Geometry: final body of the model. Coordinates: model frame, mm. A direction names the side the tool comes from. Coordinates: 2 decimals unless noted, no trailing zeros. Order: outer loops, then holes, each group sorted by start corner. A loop starts at its lowest first (then second) coordinate and runs counter-clockwise, first axis right, second up. Notation, with made-up numbers: (54, -32.5) - (111, -32.5) arc R28 cw to (111, -2.5) - close; hole circle Ø5 at (66, 39.25). An arc over 180 degrees is marked (long way). Use a Markdown table: item, result. Add a question column.
```python
from build123d import *

# Parameters (mm, degrees)
SKETCH1_W           = 160
SKETCH1_H           = 120
BOSS_EXTRUDE1_DEPTH = 3
SKETCH2_W           = 160
SKETCH2_H           = 120
SKETCH2_W_2         = 148
SKETCH2_H_2         = 116
BOSS_EXTRUDE2_DEPTH = 50
SKETCH3_R           = 1
CUT_EXTRUDE1_DEPTH  = 179.910592196
SKETCH4_R           = 1.6
SKETCH4_R_2         = 2.6
SKETCH4_R_3         = 1.4
CUT_EXTRUDE2_DEPTH  = 173.678892746
SKETCH5_W           = 5.5
SKETCH5_H           = 5.5
NUT_CAVITIES_DEPTH  = 2.5
CUT_EXTRUDE3_DEPTH  = 10


with BuildPart() as part:
    # Sketch1 → Boss-Extrude1 (new body)
    with BuildSketch(Plane(origin=(0, 0, 0), x_dir=(1, 0, 0), z_dir=(0, 1, 0))):
        Rectangle(SKETCH1_W, SKETCH1_H)
    extrude(amount=BOSS_EXTRUDE1_DEPTH)

    # Sketch2 → Boss-Extrude2 (add)
    with BuildSketch(Plane(origin=(0, 3, 0), x_dir=(1, 0, 0), z_dir=(0, 1, 0))):
        Rectangle(SKETCH2_W, SKETCH2_H)
        with Locations((-1, 0)):
            Rectangle(SKETCH2_W_2, SKETCH2_H_2, mode=Mode.SUBTRACT)
    extrude(amount=BOSS_EXTRUDE2_DEPTH)

    # Sketch3 → Cut-Extrude1 (cut, through all)
    with BuildSketch(Plane(origin=(80, 0, 0), x_dir=(0, 0, -1), z_dir=(1, 0, 0))):
        with Locations((-26.5, 31.5)):
            Circle(SKETCH3_R)
    extrude(amount=-CUT_EXTRUDE1_DEPTH, mode=Mode.SUBTRACT)

    # Sketch4 → Cut-Extrude2 (cut, through all)
    with BuildSketch(Plane.ZY.offset(-73)):
        with Locations((26.5, 25)):
            Circle(SKETCH4_R)
        with Locations((32.129165125, 34.75)):
            Circle(SKETCH4_R)
        with Locations((20.870834875, 34.75)):
            Circle(SKETCH4_R)
        with Locations((26.5, 31.5)):
            Circle(SKETCH4_R_2)
        with Locations((26.5, 47.5)):
            Circle(SKETCH4_R)
        with Locations((12.643593539, 39.5)):
            Circle(SKETCH4_R)
        with Locations((12.643593539, 23.5)):
            Circle(SKETCH4_R)
        with Locations((26.5, 15.5)):
            Circle(SKETCH4_R)
        with Locations((40.356406461, 23.5)):
            Circle(SKETCH4_R)
        with Locations((40.356406461, 39.5)):
            Circle(SKETCH4_R)
        with Locations((-22.25, 45.985571585)):
            Circle(SKETCH4_R_3)
        with Locations((-44.75, 45.985571585)):
            Circle(SKETCH4_R_3)
        with Locations((-56, 26.5)):
            Circle(SKETCH4_R_3)
        with Locations((-44.75, 7.014428415)):
            Circle(SKETCH4_R_3)
        with Locations((-22.25, 7.014428415)):
            Circle(SKETCH4_R_3)
    extrude(amount=-CUT_EXTRUDE2_DEPTH, mode=Mode.SUBTRACT)

    # Sketch5 → Nut cavities (cut)
    with BuildSketch(Plane.ZY.offset(-73)):
        with Locations((12.643593539, 39.5)):
            Rectangle(SKETCH5_W, SKETCH5_H)
        with Locations((26.5, 47.5)):
            Rectangle(SKETCH5_W, SKETCH5_H)
        with Locations((20.870834875, 34.75)):
            Rectangle(SKETCH5_W, SKETCH5_H)
        with Locations((12.643593539, 23.5)):
            Rectangle(SKETCH5_W, SKETCH5_H)
        with Locations((26.5, 15.5)):
            Rectangle(SKETCH5_W, SKETCH5_H)
        with Locations((26.5, 25)):
            Rectangle(SKETCH5_W, SKETCH5_H)
        with Locations((40.356406461, 23.5)):
            Rectangle(SKETCH5_W, SKETCH5_H)
        with Locations((32.129165125, 34.75)):
            Rectangle(SKETCH5_W, SKETCH5_H)
        with Locations((40.356406461, 39.5)):
            Rectangle(SKETCH5_W, SKETCH5_H)
    extrude(amount=-NUT_CAVITIES_DEPTH, mode=Mode.SUBTRACT)

    # Sketch8 → Cut-Extrude3 (cut)
    with BuildSketch(Plane(origin=(80, 0, 0), x_dir=(0, 0, -1), z_dir=(1, 0, 0))):
        with BuildLine():
            Line((10.5, 36.5), (10.5, 16.5))
            ThreePointArc((10.5, 16.5), (7, 13), (3.5, 16.5))
            Line((3.5, 16.5), (3.5, 36.5))
            ThreePointArc((3.5, 36.5), (7, 40), (10.5, 36.5))
        make_face()
    extrude(amount=-CUT_EXTRUDE3_DEPTH, mode=Mode.SUBTRACT)


solid = part.part
```
1) Line query: line 1 (Y direction, x = 76.9, z = 26.5); line 2 (Y direction, x = 76, z = -22); line 3 (X direction, y = 26, z = 51.5). Output: solid intervals per line, ascending. Write a range as from..to.
2) Draft query along X for faces 4 (the cylindrical face through (77.718, 38.526, 39.087)), 5 (the flat face through (-2, 28, 58)), 6 (the flat face through (80, 26, 1)). Return one class per face: released by +X, released by -X, zero draft, split by the parting line, or undercut.
3) First-contact query: pin 1 (6 mm diameter, centred on x = -21, z = -16, fed in from +Y); pin 2 (2.5 mm diameter, centred on y = 31.5, z = 26.5, fed in from +X). Flat tips, straight axial feed; report the tip coordinate or a pass-through.
4) Access query for faces 1 (the flat face through (73, 28, 1)), 2 (the flat face through (75.5, 26, 28)), 3 (the cylindrical face through (77.718, 23.57, 11.045)). Directions: +Z, -Z, +X, -X, +Y, -Y. A direction counts if a zero-diameter tool reaches every point of the face in a straight line with its end or side. Return the directions, or none.
5) Section query A-A (x = 56). Return the cut outline in (y, z).
From the geometry:
| question | item | result |
|---|---|---|
| 1 | line 1 | y = 0..13.9, 17.1..23.4, 26.6..28.9, 34.1..45.9, 49.1..53 |
| 1 | line 2 | y = 0..5.64, 8.39..44.61, 47.36..53 |
| 1 | line 3 | x = -80..-75, 73..80 |
| 2 | face 4 | zero draft |
| 2 | face 5 | undercut |
| 2 | face 6 | released by +X |
| 3 | pin 1 | stops at y = 3 |
| 3 | pin 2 | stops at x = -75 |
| 4 | face 1 | +Y |
| 4 | face 2 | none |
| 4 | face 3 | +X |
| 5 | outline | (0, -60) - (53, -60) - (53, -58) - (3, -58) - (3, 58) - (53, 58) - (53, 60) - (0, 60) - close |
